```python
from build123d import *

# Parameters (mm, degrees)
SKETCH1_R           = 1.5875
BOSS_EXTRUDE1_DEPTH = 3.175


with BuildPart() as part:
    # Sketch1 → Boss-Extrude1 (new body)
    with BuildSketch(Plane(origin=(0, 0, 0), x_dir=(1, 0, 0), z_dir=(0, 1, 0))):
        with BuildLine():
            Line((-31.4325, 33.02), (31.4325, 33.02))
            ThreePointArc((31.4325, 33.02), (32.555032015, 32.555032015), (33.02, 31.4325))
            Line((33.02, 31.4325), (33.02, -31.4325))
            ThreePointArc((33.02, -31.4325), (32.555032015, -32.555032015), (31.4325, -33.02))
            Line((31.4325, -33.02), (-31.4325, -33.02))
            ThreePointArc((-31.4325, -33.02), (-32.555032015, -32.555032015), (-33.02, -31.4325))
            Line((-33.02, -31.4325), (-33.02, 31.4325))
            ThreePointArc((-33.02, 31.4325), (-32.555032015, 32.555032015), (-31.4325, 33.02))
        make_face()
        with Locations(Location((-29.845, 29.845, 0), (0, 0, 270))):
            Circle(SKETCH1_R, mode=Mode.SUBTRACT)
        with Locations(Location((29.845, 29.845, 0), (0, 0, 270))):
            Circle(SKETCH1_R, mode=Mode.SUBTRACT)
        with Locations(Location((29.845, -29.845, 0), (0, 0, 270))):
            Circle(SKETCH1_R, mode=Mode.SUBTRACT)
        with Locations(Location((-29.845, -29.845, 0), (0, 0, 270))):
            Circle(SKETCH1_R, mode=Mode.SUBTRACT)
        with BuildLine():
            Line((-14.832243879, 25.4), (14.832243879, 25.4))
            ThreePointArc((14.832243879, 25.4), (16.298902637, 24.420009949), (15.954775894, 22.689967985))
            Line((15.954775894, 22.689967985), (1.122532015, 7.857724106))
            ThreePointArc((1.122532015, 7.857724106), (0, 7.392756121), (-1.122532015, 7.857724106))
            Line((-1.122532015, 7.857724106), (-15.954775894, 22.689967985))
            ThreePointArc((-15.954775894, 22.689967985), (-16.298902637, 24.420009949), (-14.832243879, 25.4))
        make_face(mode=Mode.SUBTRACT)
        Polygon((15.715448212, -17.960512242), (17.960512242, -15.715448212), (11.225320151, -8.980256121), (8.980256121, -11.225320151), align=None, mode=Mode.SUBTRACT)
        with BuildLine():
            Line((-14.832243879, -25.4), (14.832243879, -25.4))
            ThreePointArc((14.832243879, -25.4), (16.298902637, -24.420009949), (15.954775894, -22.689967985))
            Line((15.954775894, -22.689967985), (1.122532015, -7.857724106))
            ThreePointArc((1.122532015, -7.857724106), (0, -7.392756121), (-1.122532015, -7.857724106))
            Line((-1.122532015, -7.857724106), (-15.954775894, -22.689967985))
            ThreePointArc((-15.954775894, -22.689967985), (-16.298902637, -24.420009949), (-14.832243879, -25.4))
        make_face(mode=Mode.SUBTRACT)
        Polygon((-15.715448212, 17.960512242), (-8.980256121, 11.225320151), (-11.225320151, 8.980256121), (-17.960512242, 15.715448212), align=None, mode=Mode.SUBTRACT)
        Polygon((-17.960512242, -15.715448212), (-11.225320151, -8.980256121), (-8.980256121, -11.225320151), (-15.715448212, -17.960512242), align=None, mode=Mode.SUBTRACT)
        with BuildLine():
            Line((-22.689967985, 15.954775894), (-7.857724106, 1.122532015))
            ThreePointArc((-7.857724106, 1.122532015), (-7.392756121, 0), (-7.857724106, -1.122532015))
            Line((-7.857724106, -1.122532015), (-22.689967985, -15.954775894))
            ThreePointArc((-22.689967985, -15.954775894), (-24.420009949, -16.298902637), (-25.4, -14.832243879))
            Line((-25.4, -14.832243879), (-25.4, 14.832243879))
            ThreePointArc((-25.4, 14.832243879), (-24.420009949, 16.298902637), (-22.689967985, 15.954775894))
        make_face(mode=Mode.SUBTRACT)
        Polygon((-4.490128061, 2.24506403), (-2.24506403, 4.490128061), (4.490128061, -2.24506403), (2.24506403, -4.490128061), align=None, mode=Mode.SUBTRACT)
        Polygon((8.980256121, 11.225320151), (15.715448212, 17.960512242), (17.960512242, 15.715448212), (11.225320151, 8.980256121), align=None, mode=Mode.SUBTRACT)
        with BuildLine():
            Line((25.4, -14.832243879), (25.4, 14.832243879))
            ThreePointArc((25.4, 14.832243879), (24.420009949, 16.298902637), (22.689967985, 15.954775894))
            Line((22.689967985, 15.954775894), (7.857724106, 1.122532015))
            ThreePointArc((7.857724106, 1.122532015), (7.392756121, 0), (7.857724106, -1.122532015))
            Line((7.857724106, -1.122532015), (22.689967985, -15.954775894))
            ThreePointArc((22.689967985, -15.954775894), (24.420009949, -16.298902637), (25.4, -14.832243879))
        make_face(mode=Mode.SUBTRACT)
    extrude(amount=BOSS_EXTRUDE1_DEPTH)


solid = part.part
```
Can you work these out from the model? Positions are in its coordinate system, mm. Round coordinates to 2 decimals unless told otherwise and drop trailing zeros. Loops run counter-clockwise (first coordinate to the right, second up) from the corner with the lowest first, then second, coordinate; pieces in that order, holes last. Notation, with made-up numbers: M 42.25,36 L 58.25,36 A19 ccw 58.25,72 Z; hole C -2,40 d7. An arc over 180 degrees is marked long. Answer in a Markdown table with one row per item.
1. If we section it at A-A, the plane z = -6: Please give me the cut outline in (x, y) (3 decimals).
Established:
| item | result |
|---|---|
| outline | M -33.02,0 L -25.4,0 L -25.4,3.175 L -33.02,3.175 Z; M -12.735,0 L 12.735,0 L 12.735,3.175 L -12.735,3.175 Z; M 25.4,0 L 33.02,0 L 33.02,3.175 L 25.4,3.175 Z |
2. I'm going to push a flat-ended pin straight in: pin 1 Ø4 at (x, z) = (29.845, -29.845) entering from +Y (3 decimals). Where does the tip first touch, or does it pass through?
Established:
| item | result |
|---|---|
| pin 1 | y = 3.175 |
3. If we section it at D-D, the plane y = 0.6: Give the number of separate pieces and of enclosed holes in the cut face, plus the area to 3 significant figures.
Established:
| item | result |
|---|---|
| separate pieces | 1 |
| enclosed holes | 13 |
| area | 2,810 mm² |
4. Please list where these lines run through material, in increasing order: line 1 (X direction, y = 2.9, z = -30); line 2 (X direction, y = 2, z = 10); line 3 (Z direction, x = 17.5, y = 0.75). Write a range as from..to.
Established:
| item | result |
|---|---|
| line 1 | -33.02..-31.42, -28.27..28.27, 31.42..33.02 |
| line 2 | -33.02..-25.4, -16.74..-12.25, -10.21..-3.26, 3.26..10.21, 12.25..16.74, 25.4..33.02 |
| line 3 | -33.02..-16.18, -15.25..-10.76, 10.76..15.25, 16.18..33.02 |
5. Thinking about a two-plate mould opening in Z: for faces 1 (the face through (0, 2, -33.02)), 2 (the face through (-32.54, 1.57, 32.57)), 3 (the face through (-25.4, 2, 0)), which applies, pulls with the +Z half, pulls with the -Z half, needs draft (parallel to the pull), parting line crosses it, or undercut?
Established:
| item | result |
|---|---|
| face 1 | pulls with the -Z half |
| face 2 | pulls with the +Z half |
| face 3 | undercut |
6. If we section it at C-C, the plane z = -19.5: Please give me the cut outline in (x, y) (3 decimals), plus the area to 3 significant figures.
Established:
| item | result |
|---|---|
| outline | M -33.02,0 L -12.765,0 L -12.765,3.175 L -33.02,3.175 Z; M 12.765,0 L 33.02,0 L 33.02,3.175 L 12.765,3.175 Z |
| area | 129 mm² |
7. If we section it at B-B, the plane x = 21.5: Please give me the cut outline in (y, z) (3 decimals), plus the area to 3 significant figures.
Established:
| item | result |
|---|---|
| outline | M 0,-33.02 L 3.175,-33.02 L 3.175,-14.765 L 0,-14.765 Z; M 0,14.765 L 3.175,14.765 L 3.175,33.02 L 0,33.02 Z |
| area | 116 mm² |
